Solid Edge part; units mm, degrees
sketch "Sketch1" plane through (0, 0, 0) normal (0, 0, 1) x (1, 0, 0)
  circle A0 centre (35.425, -40) radius 1.7
  line L0 (11.95, -46) -> (39.95, -46)
  line L1 (39.95, -46) -> (39.95, -36)
  line L2 (11.95, -36) -> (39.95, -36)
  line L3 (11.95, -36) -> (11.95, -46)
  circle A1 centre (16.425, -40) radius 1.7
extrude "Protrusion1" add sketch "Sketch1" along normal blind 11
sketch "Sketch2" plane through (25.95, -46, 4) normal (0, -1, 0) x (-1, 0, 0)
  circle A0 centre (0, -1.5) radius 2.2
extrude "Cutout1" cut sketch "Sketch2" against normal through all
sketch "Sketch3" plane through (25.95, -41, 11) normal (0, 0, 1) x (-1, 0, 0)
  line L0 (-9.475, -1) -> (-8.2521, 0.1809)
  line L1 (-8.2521, 0.1809) -> (-9.475, 1.4472)
  line L2 (-9.475, 1.4472) -> (-10.6979, 0.1809)
  line L3 (-10.6979, 0.1809) -> (-9.475, -1)
  line L4 (9.525, -1) -> (10.7479, 0.1809)
  line L5 (10.7479, 0.1809) -> (9.525, 1.4472)
  line L6 (9.525, 1.4472) -> (8.3021, 0.1809)
  line L7 (8.3021, 0.1809) -> (9.525, -1)
extrude "Cutout2" cut sketch "Sketch3" against normal through all
extrude "ExtrudedCutout_3" [suppressed]
properties material "ABS Plastic, medium impact"
The listing builds one solid part. Answer for the finished solid, in the listing's coordinates (mm). A direction names the side the tool comes from. Round coordinates to 2 decimals unless told otherwise and drop trailing zeros. Loops run counter-clockwise (first coordinate to the right, second up) from the corner with the lowest first, then second, coordinate; pieces in that order, holes last.
1) A cutting plane is placed at D-D on y = -36.75. Determine the outline of the cut face in (x, z), plus the area to 3 significant figures.
Outcome:
outline: (11.95, 0) - (39.95, 0) - (39.95, 11) - (11.95, 11) - close; hole circle Ø4.4 at (25.95, 5.5)
area: 293 mm2
2) For a pull along X with two mould halves and no side action, classify faces 3 (the face through (11.95, -41, 5)), 4 (the face through (26, -41, 0)), 5 (the face through (15.8, -41.8, 5.6)) as released by +X, released by -X, zero draft, split by the parting line, or undercut.
Outcome:
face 3: released by -X
face 4: zero draft
face 5: undercut
3) A cutting plane is placed at B-B on z = 5.5. Give the number of separate pieces and of enclosed holes in the cut face, plus the area to 3 significant figures.
Outcome:
separate pieces: 2
enclosed holes: 2
area: 216 mm2
4) For faces 1 (the face through (34.8, -41.8, 5.6)), 2 (the face through (39.95, -41, 5)), determine the directions among +Z, -Z, +X, -X, +Y, -Y from which every point of the face is accessible in a straight line to the end or side of a thin tool.
Outcome:
face 1: +Z, -Z
face 2: +Z, -Z, +X, +Y, -Y
5) A cutting plane is placed at C-C on x = 25.95. Determine the outline of the cut face in (y, z), plus the area to 3 significant figures.
Outcome:
outline: (-46, 0) - (-36, 0) - (-36, 3.3) - (-46, 3.3) - close; (-46, 7.7) - (-36, 7.7) - (-36, 11) - (-46, 11) - close
area: 66.0 mm2
6) A cutting plane is placed at A-A on y = -40. Determine the outline of the cut face in (x, z) (3 decimals).
Outcome:
outline: (11.95, 0) - (14.725, 0) - (14.725, 11) - (11.95, 11) - close; (18.125, 0) - (33.725, 0) - (33.725, 11) - (18.125, 11) - close; (37.125, 0) - (39.95, 0) - (39.95, 11) - (37.125, 11) - close; hole circle Ø4.4 at (25.95, 5.5)
7) Consider line 1 (X direction, y = -40, z = 2.5) (3 decimals); line 2 (Z direction, x = 25.95, y = -42.25); line 3 (X direction, y = -43.75, z = 5.5). Determine where each line is inside the solid, lowest interval first.
Outcome:
line 1: x = 11.95 to 14.725, 18.125 to 33.725, 37.125 to 39.95
line 2: z = 0 to 3.3, 7.7 to 11
line 3: x = 11.95 to 23.75, 28.15 to 39.95
